from build123d import *

# Parameters (mm, degrees)
BOSS_EXTRUDE1_DEPTH = 30
SKETCH2_R           = 7.5
BOSS_EXTRUDE2_DEPTH = 20
SKETCH3_R           = 7.5
CUT_EXTRUDE1_DEPTH  = 20


with BuildPart() as part:
    # Sketch1 → Boss-Extrude1 (new body)
    with BuildSketch(Plane.XY):
        with BuildLine():
            Line((0, 0), (0, 60))
            Line((0, 60), (55, 60))
            ThreePointArc((55, 60), (70, 45), (55, 30))
            Line((55, 30), (30, 30))
            Line((30, 30), (30, -30))
            Line((30, -30), (0, 0))
        make_face()
    boss_extrude1 = extrude(amount=BOSS_EXTRUDE1_DEPTH)

    # Sketch2 → Boss-Extrude2 (add)
    with BuildSketch(Plane.XY.offset(30)):
        with Locations((55, 45)):
            Circle(SKETCH2_R)
    boss_extrude2 = extrude(amount=BOSS_EXTRUDE2_DEPTH)

    # Sketch3 → Cut-Extrude1 (cut)
    with BuildSketch(Plane(origin=(0, 60, 0), x_dir=(1, 0, 0), z_dir=(0, 1, 0))):
        with Locations(Location((15, -15, 0), (0, 0, 270))):
            Circle(SKETCH3_R)
    cut_extrude1 = extrude(amount=-CUT_EXTRUDE1_DEPTH, mode=Mode.SUBTRACT)

    # Mirror1: Boss-Extrude1, Boss-Extrude2, Cut-Extrude1 across plane
    add(boss_extrude1.mirror(Plane(origin=(30, -30, 30), x_dir=(0, 0, 1), z_dir=(0.7071067811865512, 0.7071067811865439, 0))))
    add(boss_extrude2.mirror(Plane(origin=(30, -30, 30), x_dir=(0, 0, 1), z_dir=(0.7071067811865512, 0.7071067811865439, 0))))
    add(cut_extrude1.mirror(Plane(origin=(30, -30, 30), x_dir=(0, 0, 1), z_dir=(0.7071067811865512, 0.7071067811865439, 0))), mode=Mode.SUBTRACT)


solid = part.part
Geometry check sheet. Reference: the model listing, model coordinates, mm. A direction names the side the tool comes from. Give positions to 0.01 mm unless a question says otherwise; leave off trailing zeros. Loops run counter-clockwise (first coordinate to the right, second up) from the corner with the lowest first, then second, coordinate; pieces in that order, holes last. Notation, with made-up numbers: M -36.75,89.5 L 18.25,89.5 A5 ccw 18.25,98.5 Z; hole C 4.25,60 d9. An arc over 180 degrees is marked long. Answer as a JSON object with one key per item and string values. Group by question number.
Item 1: Mould release check, pull along Z, two halves, no side actions. Record for faces 1 (the flat face through (55, 45, 50)), 2 (the flat face through (-40, -15, 15)), 3 (the flat face through (4, 9, 0)): pulls with the +Z half, pulls with the -Z half, needs draft (parallel to the pull), parting line crosses it, or undercut.
Item 2: Sectioned sample at A-A on x = -45. Record the boundary of the cut face in (y, z).
Item 3: Sectioned sample at C-C on z = 15. Record the boundary of the cut face in (x, y), plus the area to 3 significant figures.
Item 4: Gauge pin test, flat ends, axial feed: pin 1 (7.5 mm diameter, centred on y = -12.5, z = 15, fed in from -X); pin 2 (5 mm diameter, centred on x = -32.5, z = 30, fed in from -Y); pin 3 (4 mm diameter, centred on y = 19.5, z = 23.5, fed in from -X). Record the tip position at first contact, or that the pin passes through.
Item 5: Access from +Z, -Z, +X, -X, +Y, -Y to the whole of each face (thin tool, end or side, straight path). Record for faces 4 (the flat face through (-30, 0, 15)), 5 (the cylindrical face through (53.37, 37.68, 39.86)), 6 (the cylindrical face through (-50.14, -7.68, 13.37)), 7 (the cylindrical face through (21.324, 50.14, 19.032)), 8 (the flat face through (43, 30, 15)).
Item 6: Sectioned sample at D-D on z = 43. Record the boundary of the cut face in (x, y).
Item 7: Material ranges on L1, parallel to X at y = 45.25, z = 15; L2, parallel to Y at x = 30.5, z = 3; L3, parallel to Y at x = -21, z = 25.5, recorded low to high.
Item 8: Sectioned sample at B-B on y = -15. Record the boundary of the cut face in (x, z), plus the area to 3 significant figures.
Findings below:
{
 "1": {"face 1": "pulls with the +Z half", "face 2": "undercut", "face 3": "pulls with the -Z half"},
 "2": {"outline": "M -70,0 L 0,0 L 0,30 L -47.5,30 L -47.5,50 L -62.5,50 L -62.5,30 L -70,30 Z; hole C -15,15 d15"},
 "3": {"outline": "M -60,-55 A15 ccw -30,-55 L -30,-30 L 30,-30 L 30,30 L 55,30 A15 ccw 55,60 L 22.5,60 L 22.5,40 L 7.5,40 L 7.5,60 L 0,60 L 0,0 L -60,0 L -60,-7.5 L -40,-7.5 L -40,-22.5 L -60,-22.5 Z", "area": "6,110 mm2"},
 "4": {"pin 1": "x = -40", "pin 2": "y = -66.18", "pin 3": "x = 0"},
 "5": {"face 4": "+Z, -Z, -X, +Y", "face 5": "+Z", "face 6": "-X", "face 7": "+Y", "face 8": "+Z, -Z, +X, -Y"},
 "6": {"outline": "C -45,-55 d15; C 55,45 d15"},
 "7": {"L1": "0 to 7.5, 22.5 to 70", "L2": "30 to 60", "L3": "-30 to 0"},
 "8": {"outline": "M -60,0 L 30,0 L 30,30 L -60,30 L -60,22.5 L -40,22.5 L -40,7.5 L -60,7.5 Z", "area": "2,400 mm2"}
}
